Design review of the part built by this model. Coordinates are the model's own, in mm. Face numbers are marked on the shaded views. Round coordinates to 2 decimals unless told otherwise and drop trailing zeros. Write each loop counter-clockwise with the first axis right and the second up, starting at its lowest first coordinate (ties: lowest second). Pieces come first, ordered by that corner, then holes. Notation, with made-up numbers: M -3,10.5 L 12,10.5 A10 ccw 12,20.5 Z; hole C -7,53 d1. An arc over 180 degrees is marked long. One line per question, with ' | ' between items. Start each with the question number.
Item 1: Draft analysis for pull direction X (two halves, no side actions). For the marked faces 1 and 2, state which applies: released by +X, released by -X, zero draft, split by the parting line, or undercut.
Item 2: Add section D-D, the plane x = -17. State the section outline as (y, z) points, and give its area (3 significant figures).
Item 3: Add section C-C, the plane z = 1.5. State the section outline as (x, y) points, and give its area (3 significant figures).
Item 4: Insertion check: pin 1 Ø1.5 at (x, y) = (-95.5, 7) entering from +Z; pin 2 Ø1.5 at (y, z) = (6.5, -12.5) entering from +X; pin 3 Ø1.5 at (y, z) = (6, -9) entering from -X. Each pin has a flat end and moves straight along its axis. Give the tip position at first contact, or say it passes through.
Item 5: Add section B-B, the plane x = -82. State the section outline as (y, z) points.
Item 6: For L1, parallel to X at y = 5.25, z = 28.5; L2, parallel to Z at x = -145, y = 7.25; L3, parallel to Y at x = 141, z = -33, list the stretches that pass through material, from the lowest coordinate up.
Item 7: Add section A-A, the plane y = 6.5. State the section outline as (x, z) points, and give its area (3 significant figures).
```python
from build123d import *

# Parameters (mm, degrees)
SKETCH2_W           = 350
SKETCH2_H           = 350
BOSS_EXTRUDE1_DEPTH = 5
SKETCH4_W           = 90.2
SKETCH4_H           = 90.2
BOSS_EXTRUDE2_DEPTH = 3


with BuildPart() as part:
    # Sketch2 → Boss-Extrude1 (new body)
    with BuildSketch(Plane(origin=(0, 0, 0), x_dir=(1, 0, 0), z_dir=(0, 1, 0))):
        Rectangle(SKETCH2_W, SKETCH2_H)
    extrude(amount=BOSS_EXTRUDE1_DEPTH)

    # Sketch4 → Boss-Extrude2 (add)
    with BuildSketch(Plane(origin=(0, 5, 0), x_dir=(1, 0, 0), z_dir=(0, 1, 0))):
        Polygon((-56.121208512, 45.1), (-56.121208512, 48.622803372), (-59.9, 48.622803372), (-150.1, 48.622803372), (-153.264875212, 48.622803372), (-153.264875212, 45.1), (-153.264875212, -45.1), (-153.264875212, -48.557517283), (-150.1, -48.557517283), (-59.9, -48.557517283), (-56.121208512, -48.557517283), (-56.121208512, -45.1), align=None)
        with Locations((-105, 0)):
            Rectangle(SKETCH4_W, SKETCH4_H, mode=Mode.SUBTRACT)
    extrude(amount=BOSS_EXTRUDE2_DEPTH)


solid = part.part
```
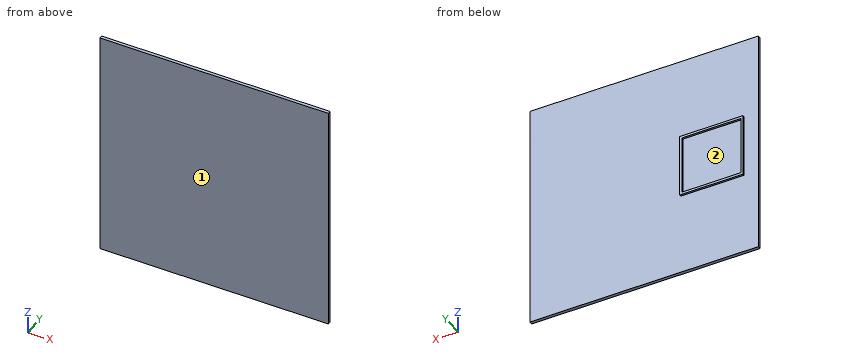
Computed values:
1) face 1: zero draft | face 2: undercut
2) outline: M 0,-175 L 5,-175 L 5,175 L 0,175 Z | area: 1,750 mm^2
3) outline: M -175,0 L 175,0 L 175,5 L -56.12,5 L -56.12,8 L -59.9,8 L -59.9,5 L -150.1,5 L -150.1,8 L -153.26,8 L -153.26,5 L -175,5 Z | area: 1,770 mm^2
4) pin 1: stops at z = 48.56 | pin 2: stops at x = -56.12 | pin 3: stops at x = -153.26
5) outline: M 0,-175 L 5,-175 L 5,-48.62 L 8,-48.62 L 8,-45.1 L 5,-45.1 L 5,45.1 L 8,45.1 L 8,48.56 L 5,48.56 L 5,175 L 0,175 Z
6) L1: x = -153.26 to -150.1, -59.9 to -56.12 | L2: z = -48.62 to -45.1, 45.1 to 48.56 | L3: y = 0 to 5
7) outline: M -153.26,-48.62 L -56.12,-48.62 L -56.12,48.56 L -153.26,48.56 Z; hole M -150.1,-45.1 L -59.9,-45.1 L -59.9,45.1 L -150.1,45.1 Z | area: 1,300 mm^2
